```python
from build123d import *

# Parameters (mm, degrees)
SKETCH1_R           = 11.735
BOSS_EXTRUDE1_DEPTH = 17.64
SKETCH2_R           = 13.44
BOSS_EXTRUDE2_DEPTH = 4
SKETCH3_R           = 9.705
BOSS_EXTRUDE3_DEPTH = 4.62
FILLET1_R           = 4
FILLET2_R           = 0.5
SKETCH4_W           = 0.5
SKETCH4_H           = 2.67
BOSS_EXTRUDE4_DEPTH = 7.51


with BuildPart() as part:
    # Sketch1 → Boss-Extrude1 (new body)
    with BuildSketch(Plane(origin=(0, 0, 0), x_dir=(1, 0, 0), z_dir=(0, 1, 0))):
        with Locations(Location((0, 0, 0), (0, 0, 270))):
            Circle(SKETCH1_R)
    extrude(amount=BOSS_EXTRUDE1_DEPTH)

    # Sketch2 → Boss-Extrude2 (add)
    with BuildSketch(Plane(origin=(0, 17.64, 0), x_dir=(1, 0, 0), z_dir=(0, 1, 0))):
        with Locations(Location((0, 0, 0), (0, 0, 270))):
            Circle(SKETCH2_R)
    extrude(amount=BOSS_EXTRUDE2_DEPTH)

    # Sketch3 → Boss-Extrude3 (add)
    with BuildSketch(Plane(origin=(0, 21.64, 0), x_dir=(1, 0, 0), z_dir=(0, 1, 0))):
        with Locations(Location((0, 0, 0), (0, 0, 270))):
            Circle(SKETCH3_R)
    extrude(amount=BOSS_EXTRUDE3_DEPTH)

    # Fillet1
    # the kernel refuses this fillet: 4 mm, written as the material it takes off along each edge
    with BuildSketch(Plane(origin=(0, 21.64, 0), x_dir=(0, 0, 1), z_dir=(-1, 0, 0))) as fillet1_piece_1:
        with BuildLine():
            CenterArc((9.44, -3.991212222), FILLET1_R, 0, 86.201372408)
            Line((9.705, 0), (9.7103, 0.079824244))
            ThreePointArc((9.7103, 0.079824244), (11.5725, 0.08), (13.44, 0.08))
            Line((13.44, 0.08), (13.52, 0))
            Line((13.52, 0), (13.52, -3.991212222))
            Line((13.52, -3.991212222), (13.44, -3.991212222))
        make_face()
    revolve(axis=Axis((0, 21.64, 0), (0, 1, 0)), mode=Mode.SUBTRACT)

    # Fillet2
    fillet2_edges = [part.edges().sort_by_distance(p)[0] for p in [
        (0, 26.26, -9.705),
    ]]
    fillet(fillet2_edges, radius=FILLET2_R)

    # Sketch4 → Boss-Extrude4 (add)
    with BuildSketch(Plane.XZ):
        with Locations((6.45, 3.27)):
            Rectangle(SKETCH4_W, SKETCH4_H)
        with Locations((6.45, -3.275)):
            Rectangle(SKETCH4_W, SKETCH4_H)
    extrude(amount=BOSS_EXTRUDE4_DEPTH)


solid = part.part
```
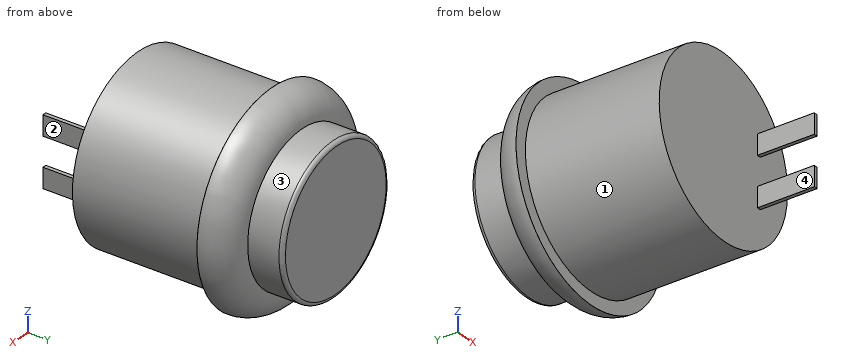
CAD build for the part. Positions are in the model's coordinates, mm. Face numbers are marked on the shaded views. A direction names the side the tool comes from. Round coordinates to 2 decimals unless told otherwise and drop trailing zeros. Order: outer loops, then holes, each group sorted by start corner. A loop starts at its lowest first (then second) coordinate and runs counter-clockwise, first axis right, second up. Notation, with made-up numbers: (-31, -19) - (13, -19) arc R13 cw to (13, 4) - close; hole circle Ø10 at (-23, -39.5). An arc over 180 degrees is marked (long way). Answer as CSV lines item,"result". Start each with the question number.
1. Saw through at B-B, the plane x = 0. Write the cut outline in (y, z) (3 decimals).
2. Tool access for the marked faces 1, 2, 3 and 4: list every direction of +Z, -Z, +X, -X, +Y, -Y with a clear straight run to the whole face (end or side of a thin tool).
3. Drill centre lines: L1, parallel to Y at x = 4, z = -1.5; L2, parallel to X at y = 2, z = 0.25; L3, parallel to X at y = -4, z = 4.25. Where is each one in solid material? Low to high. Write a range as [from, to].
4. Saw through at A-A, the plane z = 0. Write the cut outline in (x, y) (3 decimals).
5. Pin check, flat tips, straight feed: pin 1 (4 mm diameter, centred on y = -3.5, z = 1, fed in from +X); pin 2 (3 mm diameter, centred on x = 6, y = 4, fed in from +Z); pin 3 (0.6 mm diameter, centred on x = 6.5, y = -3.5, fed in from -Z). Stop position of each tip, or through.
6. Saw through at C-C, the plane y = 3.5. Write the cut outline in (x, z) (3 decimals).
Model answer:
1,outline,"(0, -11.735) - (17.64, -11.735) - (17.64, -13.44) - (17.649, -13.44) arc R4 ccw to (21.64, -9.705) - (25.76, -9.705) arc R0.5 ccw to (26.26, -9.205) - (26.26, 9.205) arc R0.5 ccw to (25.76, 9.705) - (21.64, 9.705) arc R4 ccw to (17.649, 13.44) - (17.64, 13.44) - (17.64, 11.735) - (0, 11.735) - close"
2,face 1,"-Y"
2,face 2,"+Z, -Z, +X, -Y"
2,face 3,"+Y"
2,face 4,"+Z, -Z, -X, -Y"
3,L1,"y = [0, 26.26]"
3,L2,"x = [-11.73, 11.73]"
3,L3,"x = [6.2, 6.7]"
4,outline,"(-13.44, 17.64) - (-11.735, 17.64) - (-11.735, 0) - (11.735, 0) - (11.735, 17.64) - (13.44, 17.64) - (13.44, 17.649) arc R4 ccw to (9.705, 21.64) - (9.705, 25.76) arc R0.5 ccw to (9.205, 26.26) - (-9.205, 26.26) arc R0.5 ccw to (-9.705, 25.76) - (-9.705, 21.64) arc R4 ccw to (-13.44, 17.649) - close"
5,pin 1,"stops at x = 6.7"
5,pin 2,"stops at z = 10.84"
5,pin 3,"stops at z = -4.61"
6,outline,"circle Ø23.47 at (0, 0)"
